Check sheet for the modelled part. Datum: model origin and axes. Units: mm. Coordinates: 2 decimals unless noted, no trailing zeros. Order: outer loops, then holes, each group sorted by start corner. A loop starts at its lowest first (then second) coordinate and runs counter-clockwise, first axis right, second up.
1. Cross-section at C-C (z = 35). Enter the section's corners in (x, y), then the cut area to 3 significant figures.
2. Thickness scan on line 1 (Z direction, x = 0, y = -30.75); line 2 (Y direction, x = 0, z = 38); line 3 (Y direction, x = 11.5, z = 10). Record the ranges inside material, lowest first.
3. Cross-section at A-A (y = 0). Enter the section's corners in (x, z), then the cut area to 4 significant figures.
4. Draft check along Z on faces 1 (the cylindrical face through (-3, -30, 10)), 2 (the flat face through (17, -17, 105)), 3 (the flat face through (17, -17, 0)). Enter one of: released by +Z, released by -Z, zero draft, split by the parting line, or undercut.
5. Cross-section at B-B (x = 0). Enter the section's corners in (y, z).
6. Gauge pin test, flat ends, axial feed: pin 1 Ø6 at (y, z) = (4.5, 54) entering from +X; pin 2 Ø10 at (x, z) = (2.5, 89.5) entering from +Y; pin 3 Ø3 at (y, z) = (-19.5, 75) entering from +X; pin 4 Ø8 at (x, z) = (0, 10) entering from -Y. Record the tip position at first contact, or that the pin passes through.
7. Cross-section at D-D (y = -34). Enter the section's corners in (x, z).
```python
from build123d import *

# Parameters (mm, degrees)
F0_R     = 40
F1_DEPTH = 105
F2_R     = 20.5
F3_DEPTH = 105.001
F4_R     = 3
F5_DEPTH = 40.001


with BuildPart() as f1:
    # F0 (on Top) → F1 (new body)
    with BuildSketch(Plane.XY):
        Circle(F0_R)
    extrude(amount=F1_DEPTH)

    # F2 (on face) → F3 (cut, through all)
    with BuildSketch(Plane.XY.offset(105)):
        Circle(F2_R)
    extrude(amount=-F3_DEPTH, mode=Mode.SUBTRACT)

    # F4 (on Front) → F5 (cut, through all)
    with BuildSketch(Plane.XZ):
        with Locations((0, 10)):
            Circle(F4_R)
    extrude(amount=F5_DEPTH, mode=Mode.SUBTRACT)


solid = f1.part
```
Data:
1. outline: circle Ø80 at (0, 0); hole circle Ø41 at (0, 0)
1. area: 3,710 mm2
2. line 1: z = 0 to 7, 13 to 105
2. line 2: y = -40 to -20.5, 20.5 to 40
2. line 3: y = -38.31 to -16.97, 16.97 to 38.31
3. outline: (-40, 0) - (-20.5, 0) - (-20.5, 105) - (-40, 105) - close; (20.5, 0) - (40, 0) - (40, 105) - (20.5, 105) - close
3. area: 4,095 mm2
4. face 1: undercut
4. face 2: released by +Z
4. face 3: released by -Z
5. outline: (-40, 0) - (-20.5, 0) - (-20.5, 7) - (-40, 7) - close; (-40, 13) - (-20.5, 13) - (-20.5, 105) - (-40, 105) - close; (20.5, 0) - (40, 0) - (40, 105) - (20.5, 105) - close
6. pin 1: stops at x = 39.97
6. pin 2: stops at y = 40
6. pin 3: stops at x = 35.72
6. pin 4: stops at y = -40
7. outline: (-21.07, 0) - (21.07, 0) - (21.07, 105) - (-21.07, 105) - close; hole circle Ø6 at (0, 10)
